Read the model definition and answer for the solid it produces. Units are mm, in the model's axes. A direction names the side the tool comes from. Coordinates: 2 decimals unless noted, no trailing zeros. Write each loop counter-clockwise with the first axis right and the second up, starting at its lowest first coordinate (ties: lowest second). Pieces come first, ordered by that corner, then holes. Notation, with made-up numbers: (-17.5, 11) -> (-12.5, 11) arc R26 ccw to (-12.5, 46) -> close; hole circle Ø4 at (63.5, 4.5). An arc over 180 degrees is marked (long way). Answer as a JSON object with one key per item and string values. Group by question number.
(1) Straight lines are drawn through the part: L1, parallel to X at y = 7.75, z = -22.5; L2, parallel to Z at x = 3.5, y = 3.75. For each, find the intervals that lie inside material, in ascending order.
(2) Find section C-C (x = 12). Give the vertices of the cut face in (y, z).
(3) For a pull along X with two mould halves and no side action, classify faces 6 (the face through (0, 4, -11)), 7 (the face through (17, 4, -11)), 8 (the face through (8, 0, -12)), 9 (the face through (0.5, 4, -22)) as +X half, -X half, draft (parallel to the pull), parting line (faces both ways), or undercut.
(4) Find section D-D (x = 6.25). Give the vertices of the cut face in (y, z), then the cut area to 3 significant figures.
(5) Find section A-A (y = 3.5). Give the vertices of the cut face in (x, z), then the cut area to 3 significant figures.
(6) Find section B-B (z = -20.75). Give the vertices of the cut face in (x, y).
(7) Which of the six approach directions +Z, -Z, +X, -X, +Y, -Y give full straight-line access (tool end or side, diameter ignored) to faces 1 (the face through (16.8, 2.5, -23)), 2 (the face through (8, 0.5, -22)), 3 (the face through (8, 8, -9)), 4 (the face through (0.3, 3.1, -23)), 5 (the face through (8, 4, 0))?
(8) Flat-ended cylindrical pins translate along their axes: P1, Ø6, axis at x = 9.5, z = -3.5, coming from the -Y side; P2, Ø2, axis at x = 10.5, y = 4, coming from the -Z side; P3, Ø3.5, axis at x = 2, y = 4, coming from the -Z side; P4, Ø2.5, axis at x = 11, z = -22.5, coming from the +Y side. Find the tip coordinate at first contact, or state that the pin passes through.
from build123d import *

# Parameters (mm, degrees)
SKETCH_1_W      = 17
SKETCH_1_H      = 23
EXTRUDE_1_DEPTH = 0.5
SKETCH_2_W      = 0.5
SKETCH_2_H      = 23
EXTRUDE_2_DEPTH = 7.5
SKETCH_3_W      = 16
SKETCH_3_H      = 20.172343548
EXTRUDE_3_DEPTH = 7.5
SKETCH_4_W      = 2.493920062
SKETCH_4_H      = 0.457616149
SKETCH_4_W_2    = 2.364028392
EXTRUDE_4_DEPTH = 0.5


with BuildPart() as part:
    # 草图1 → 凸台-拉伸1 (new body)
    with BuildSketch(Plane(origin=(0, 0, 0), x_dir=(1, 0, 0), z_dir=(0, 1, 0))):
        with Locations((8.5, 11.5)):
            Rectangle(SKETCH_1_W, SKETCH_1_H)
    extrude(amount=EXTRUDE_1_DEPTH)

    # 草图2 → 凸台-拉伸2 (add)
    with BuildSketch(Plane(origin=(0, 0.5, 0), x_dir=(1, 0, 0), z_dir=(0, 1, 0))):
        with Locations((0.25, 11.5)):
            Rectangle(SKETCH_2_W, SKETCH_2_H)
        with Locations((16.75, 11.5)):
            Rectangle(SKETCH_2_W, SKETCH_2_H)
    extrude(amount=EXTRUDE_2_DEPTH)

    # 草图3 → 凸台-拉伸3 (add)
    with BuildSketch(Plane(origin=(0, 0.5, 0), x_dir=(1, 0, 0), z_dir=(0, 1, 0))):
        with Locations((8.5, 10.086171774)):
            Rectangle(SKETCH_3_W, SKETCH_3_H)
    extrude(amount=EXTRUDE_3_DEPTH)

    # 草图4 → 凸台-拉伸4 (add)
    with BuildSketch(Plane(origin=(0, 0.5, 0), x_dir=(1, 0, 0), z_dir=(0, 1, 0))):
        with Locations((4.291509895, 23.228808075)):
            Rectangle(SKETCH_4_W, SKETCH_4_H)
        with Locations((11.968107586, 23.228808075)):
            Rectangle(SKETCH_4_W_2, SKETCH_4_H)
    extrude(amount=-EXTRUDE_4_DEPTH)


solid = part.part
Results below:
{
 "1": {"L1": "x = 0 to 0.5, 16.5 to 17", "L2": "z = -20.17 to 0"},
 "2": {"outline": "(0, -23.46) -> (0.5, -23.46) -> (0.5, -20.17) -> (8, -20.17) -> (8, 0) -> (0, 0) -> close"},
 "3": {"face 6": "-X half", "face 7": "+X half", "face 8": "draft", "face 9": "undercut"},
 "4": {"outline": "(0, -23) -> (0.5, -23) -> (0.5, -20.17) -> (8, -20.17) -> (8, 0) -> (0, 0) -> close", "area": "163 mm2"},
 "5": {"outline": "(0, -23) -> (0.5, -23) -> (0.5, -20.17) -> (16.5, -20.17) -> (16.5, -23) -> (17, -23) -> (17, 0) -> (0, 0) -> close", "area": "346 mm2"},
 "6": {"outline": "(0, 0) -> (17, 0) -> (17, 8) -> (16.5, 8) -> (16.5, 0.5) -> (0.5, 0.5) -> (0.5, 8) -> (0, 8) -> close"},
 "7": {"face 1": "-Z, +X, +Y, -Y", "face 2": "-Z, +Y", "face 3": "+Z, -Z, +X, -X, +Y", "face 4": "-Z, -X, +Y, -Y", "face 5": "+Z, +X, -X, +Y, -Y"},
 "8": {"P1": "stops at y = 0", "P2": "stops at z = -20.17", "P3": "stops at z = -23", "P4": "stops at y = 0.5"}
}
